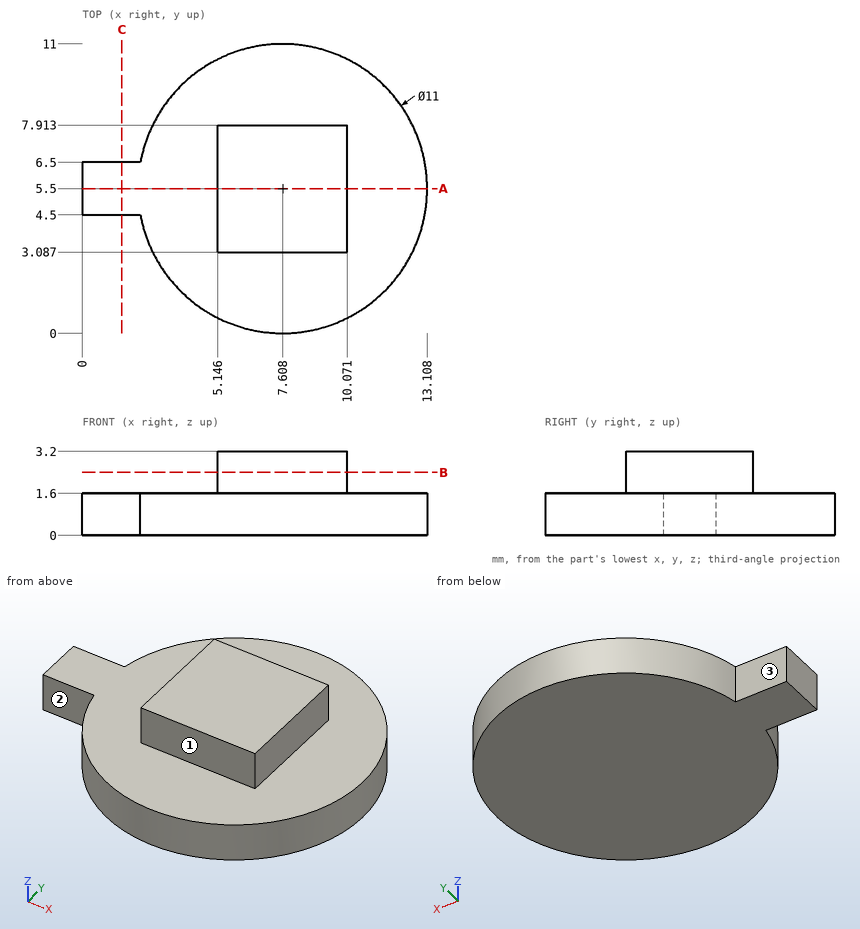
Study the drawing (mm; zero at the part's minimum x, y, z) and answer. A direction names the side the tool comes from. Round coordinates to 2 decimals unless told otherwise and drop trailing zeros. Loops run counter-clockwise (first coordinate to the right, second up) from the corner with the lowest first, then second, coordinate; pieces in that order, holes last. Notation, with made-up numbers: (81.5, 63) -> (110.5, 63) arc R18 cw to (110.5, 93) -> close; hole circle Ø9 at (40, 30). An arc over 180 degrees is marked (long way). Use one line per item in the form item = value.
1. Find the intervals of material crossed by probe 1 along Z at (x, y) = (11.25, 3.75); probe 2 along X at (y, z) = (4.5, 1.65) (1 decimal); probe 3 along Y at (x, z) = (9.75, 2.6), in increasing order. Write a range as [from, to].
Answer key:
probe_1 = [0, 1.6]
probe_2 = [5.1, 10.1]
probe_3 = [3.09, 7.91]
2. A tool of negligible diameter and unlimited length cuts with its end or side. For the marked faces 1, 2 and 3, from which of +Z, -Z, +X, -X, +Y, -Y can it reach the whole face along a straight path? Write none if from no direction.
Answer key:
face_1 = +Z, +X, -X, -Y
face_2 = +Z, -Z, -X, -Y
face_3 = +Z, -Z, -X, +Y
3. Flat-ended cylindrical pins translate along their axes: pin 1 Ø0.8 at (y, z) = (6, 2.5) entering from +X; pin 2 Ø0.8 at (x, z) = (0.5, 1) entering from -Y; pin 3 Ø1.3 at (x, z) = (1, 0.5) entering from +Y. Find the tip coordinate at first contact, or state that the pin passes through.
Answer key:
pin_1 = 10.07
pin_2 = 4.5
pin_3 = 6.5
4. The part is cut by section C-C on x = 1.5. Determine the outline of the cut face in (y, z).
Answer key:
outline = (4.5, 0) -> (6.5, 0) -> (6.5, 1.6) -> (4.5, 1.6) -> close
5. The part is cut by section B-B on z = 2.4. Determine the outline of the cut face in (x, y) (1 decimal).
Answer key:
outline = (5.1, 3.1) -> (10.1, 3.1) -> (10.1, 7.9) -> (5.1, 7.9) -> close
6. The part is cut by section A-A on y = 5.5. Determine the outline of the cut face in (x, z) (1 decimal).
Answer key:
outline = (0, 0) -> (13.1, 0) -> (13.1, 1.6) -> (10.1, 1.6) -> (10.1, 3.2) -> (5.1, 3.2) -> (5.1, 1.6) -> (0, 1.6) -> close
